Can you work these out from the drawing? Everything is in mm from the part's minimum corner. Coordinates: 2 decimals unless noted, no trailing zeros. Write each loop counter-clockwise with the first axis right and the second up, starting at its lowest first coordinate (ties: lowest second). Pieces come first, ordered by that corner, then holes. Notation, with made-up numbers: (-37, 7.5) -> (-32, 7.5) arc R19 cw to (-32, 43.5) -> close; hole circle Ø1 at (-31, 45.25). An arc over 180 degrees is marked (long way). Use a Markdown table: item, result. Add a question column.
Item 1: Imagine slicing it at D-D, the plane x = 39. Write out the boundary of the cut face in (y, z), and give its area (3 significant figures).
Item 2: If we mould it in two halves opening along X, with no side actions, what happens to the marked faces 1, 2 and 3? For each: pulls with the +X half, pulls with the -X half, needs draft (parallel to the pull), parting line crosses it, or undercut.
Item 3: Imagine slicing it at A-A, the plane y = 24.9. Write out the boundary of the cut face in (x, z).
Item 4: Imagine slicing it at B-B, the plane z = 53. Write out the boundary of the cut face in (x, y), and give its area (3 significant figures).
Item 5: Will these pins go through, and if not, where does the flat tip stop? pin 1 Ø0.9 at (y, z) = (20.5, 62) entering from -X; pin 2 Ø11 at (x, y) = (36, 24) entering from -Z.
Item 6: Imagine slicing it at C-C, the plane x = 51.75. Write out the boundary of the cut face in (y, z).
Item 7: If I drill on line 1 along Z through (x, y) = (21.75, 12); line 2 along X through (y, z) = (35.5, 53); line 3 along X through (y, z) = (26.5, 53), over which ranges is the centre line in solid material (lowest first)? Write a range as from..to.
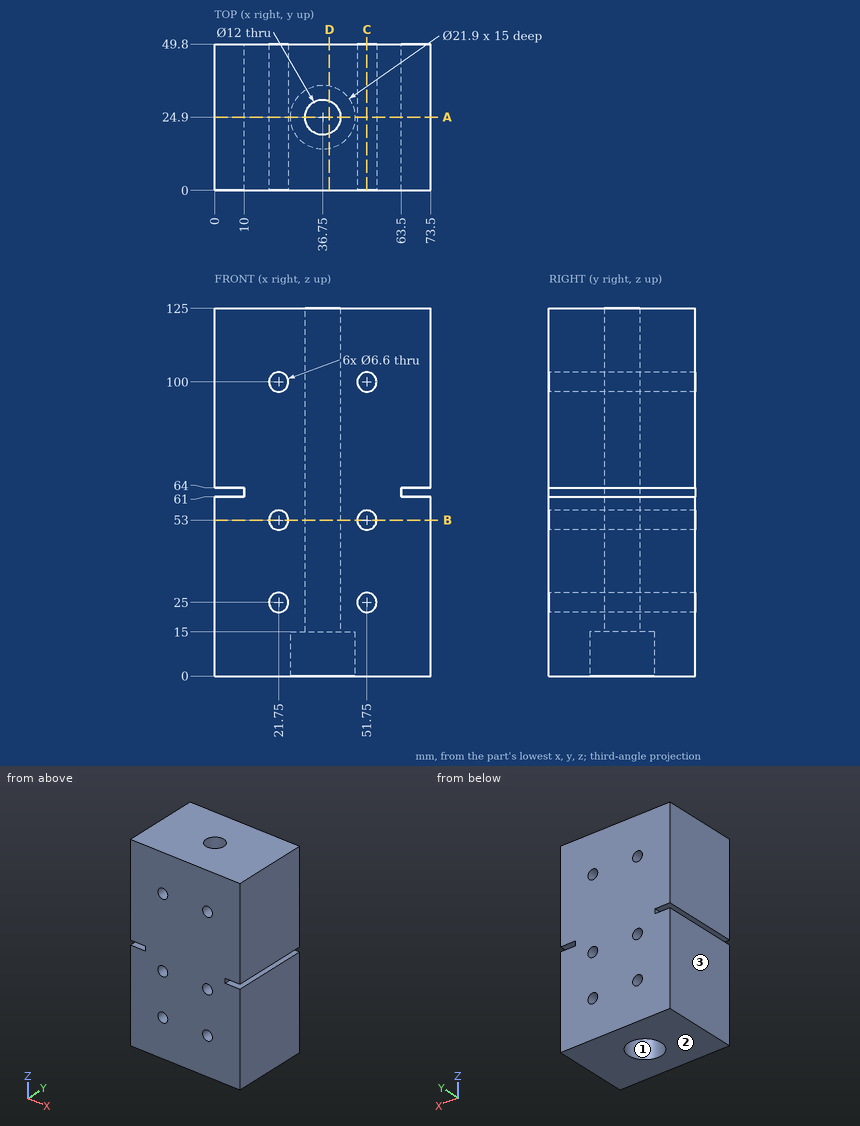
Ans:
| question | item | result |
|---|---|---|
| 1 | outline | (0, 0) -> (14.18, 0) -> (14.18, 15) -> (19.34, 15) -> (19.34, 125) -> (0, 125) -> close; (30.46, 15) -> (35.62, 15) -> (35.62, 0) -> (49.8, 0) -> (49.8, 125) -> (30.46, 125) -> close |
| 1 | area | 4,680 mm^2 |
| 2 | face 1 | undercut |
| 2 | face 2 | needs draft |
| 2 | face 3 | pulls with the -X half |
| 3 | outline | (0, 0) -> (25.8, 0) -> (25.8, 15) -> (30.75, 15) -> (30.75, 125) -> (0, 125) -> (0, 64) -> (10, 64) -> (10, 61) -> (0, 61) -> close; (42.75, 15) -> (47.7, 15) -> (47.7, 0) -> (73.5, 0) -> (73.5, 61) -> (63.5, 61) -> (63.5, 64) -> (73.5, 64) -> (73.5, 125) -> (42.75, 125) -> close; hole circle Ø6.6 at (21.75, 25); hole circle Ø6.6 at (21.75, 53); hole circle Ø6.6 at (21.75, 100); hole circle Ø6.6 at (51.75, 25); hole circle Ø6.6 at (51.75, 53); hole circle Ø6.6 at (51.75, 100) |
| 4 | outline | (0, 0) -> (18.45, 0) -> (18.45, 49.8) -> (0, 49.8) -> close; (25.05, 0) -> (48.45, 0) -> (48.45, 49.8) -> (25.05, 49.8) -> close; (55.05, 0) -> (73.5, 0) -> (73.5, 49.8) -> (55.05, 49.8) -> close; hole circle Ø12 at (36.75, 24.9) |
| 4 | area | 2,890 mm^2 |
| 5 | pin 1 | stops at x = 10 |
| 5 | pin 2 | stops at z = 15 |
| 6 | outline | (0, 0) -> (49.8, 0) -> (49.8, 21.7) -> (0, 21.7) -> close; (0, 28.3) -> (49.8, 28.3) -> (49.8, 49.7) -> (0, 49.7) -> close; (0, 56.3) -> (49.8, 56.3) -> (49.8, 96.7) -> (0, 96.7) -> close; (0, 103.3) -> (49.8, 103.3) -> (49.8, 125) -> (0, 125) -> close |
| 7 | line 1 | z = 0..21.7, 28.3..49.7, 56.3..96.7, 103.3..125 |
| 7 | line 2 | x = 0..18.45, 25.05..48.45, 55.05..73.5 |
| 7 | line 3 | x = 0..18.45, 25.05..30.97, 42.53..48.45, 55.05..73.5 |
